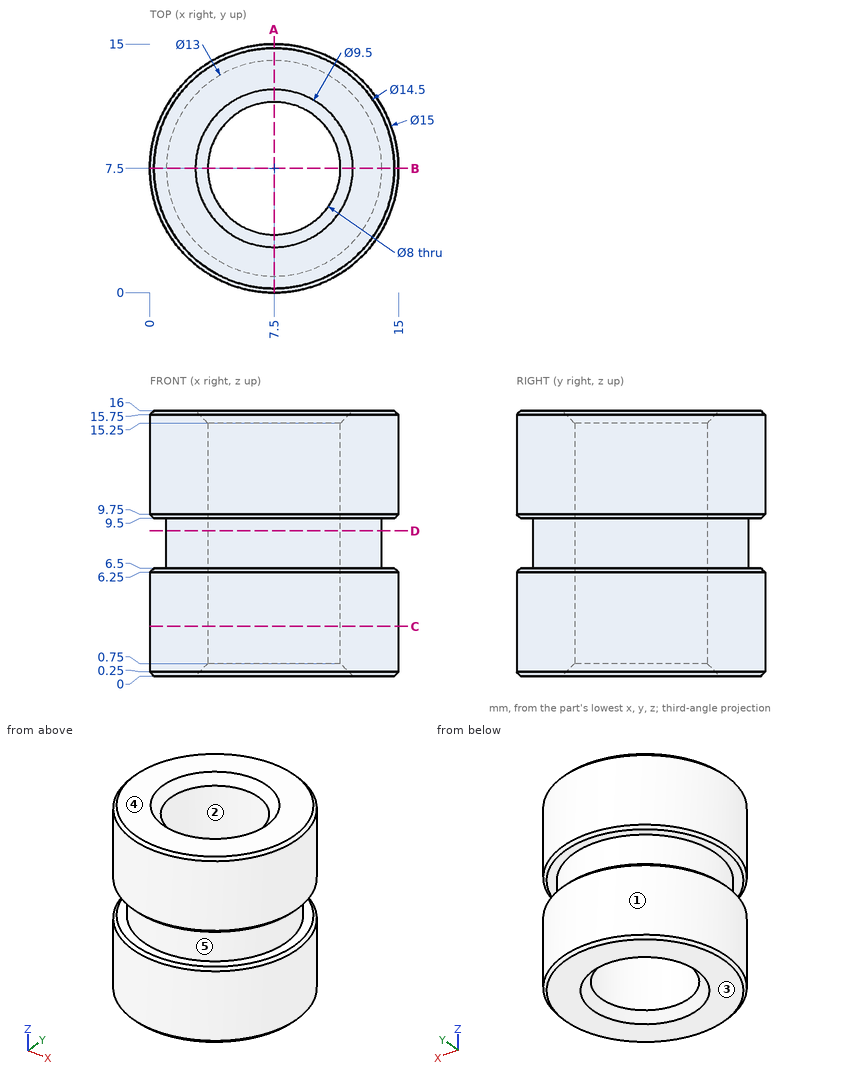
Drawing for the job (mm, zero at the part's lowest x, y, z). A direction names the side the tool comes from. Round coordinates to 2 decimals unless told otherwise and drop trailing zeros. Write each loop counter-clockwise with the first axis right and the second up, starting at its lowest first coordinate (ties: lowest second). Pieces come first, ordered by that corner, then holes. Notation, with made-up numbers: M -22,49 L -11,49 A7 ccw -11,59 Z; hole C -17,58.25 d11. An arc over 180 degrees is marked long. Answer as a JSON object with one key per item and string values. Group by question number.
(1) Mould opens along X. For the marked faces 1, 2 and 3 say: pulls with the +X half, pulls with the -X half, needs draft (parallel to the pull), parting line crosses it, or undercut.
(2) Flat gauge pins, fed straight in: pin 1 (4 mm diameter, centred on x = 2.5, z = 2, fed in from -Y); pin 2 (5 mm diameter, centred on x = 4, z = 11, fed in from -Y); pin 3 (6.5 mm diameter, centred on x = 7.5, y = 7.5, fed in from +Z); pin 4 (3 mm diameter, centred on x = 2, z = 9, fed in from +Y). Where does each tip first touch, or does it go through?
(3) Cut at D-D (z = 8.75). Give the cut face in (x, y).
(4) Drill centre lines: L1, parallel to Y at x = 7.5, z = 4.25; L2, parallel to Z at x = 6.25, y = 0.5; L3, parallel to X at y = 8.5, z = 3. Where is each one in solid material? Low to high.
(5) Which spindle directions (+Z, -Z, +X, -X, +Y, -Y) get a long thin tool onto all of the face, cutting with end or side? Do the marked faces 4 and 5. Say none if no direction does.
(6) Cut at A-A (x = 7.5). Give the cut face in (y, z), and give its area (3 significant figures).
(7) Cut at C-C (z = 3). Give the cut face in (x, y), and give its area (3 significant figures).
Responses:
{
 "1": {"face 1": "parting line crosses it", "face 2": "undercut", "face 3": "needs draft"},
 "2": {"pin 1": "stops at y = 0.63", "pin 2": "stops at y = 0.07", "pin 3": "passes through", "pin 4": "stops at y = 13.71"},
 "3": {"outline": "C 7.5,7.5 d13; hole C 7.5,7.5 d8"},
 "4": {"L1": "y = 0 to 3.5, 11.5 to 15", "L2": "z = 0 to 6.5, 9.5 to 16", "L3": "x = 0.07 to 3.63, 11.37 to 14.93"},
 "5": {"face 4": "+Z, +X, -X, +Y, -Y", "face 5": "none"},
 "6": {"outline": "M 0,0.25 L 0.25,0 L 2.75,0 L 3.5,0.75 L 3.5,15.25 L 2.75,16 L 0.25,16 L 0,15.75 L 0,9.75 L 0.25,9.5 L 1,9.5 L 1,6.5 L 0.25,6.5 L 0,6.25 Z; M 11.5,0.75 L 12.25,0 L 14.75,0 L 15,0.25 L 15,6.25 L 14.75,6.5 L 14,6.5 L 14,9.5 L 14.75,9.5 L 15,9.75 L 15,15.75 L 14.75,16 L 12.25,16 L 11.5,15.25 Z", "area": "105 mm2"},
 "7": {"outline": "C 7.5,7.5 d15; hole C 7.5,7.5 d8", "area": "126 mm2"}
}
